```python
from build123d import *

# Parameters (mm, degrees)
SKETCH_1_W          = 7
SKETCH_1_H          = 7
EXTRUDE_1_DEPTH     = 51
SKETCH_2_W          = 3.5
SKETCH_2_H          = 7
EXTRUDE_2_DEPTH     = 7
SKETCH_3_W          = 3.5
SKETCH_3_H          = 7
EXTRUDE_3_DEPTH     = 7
FILLET_1_R          = 3.5
SKETCH_4_R          = 1.55
CUT_EXTRUDE_1_DEPTH = 3.5
CUT_EXTRUDE_2_DEPTH = 3.5
FILLET_2_R          = 2


with BuildPart() as part:
    # 草图1 → 凸台-拉伸1 (new body)
    with BuildSketch(Plane.XY):
        Rectangle(SKETCH_1_W, SKETCH_1_H)
    extrude(amount=EXTRUDE_1_DEPTH)

    # 草图2 → 凸台-拉伸2 (add)
    with BuildSketch(Plane.XY.offset(51)):
        with Locations((1.75, 0)):
            Rectangle(SKETCH_2_W, SKETCH_2_H)
    extrude(amount=EXTRUDE_2_DEPTH)

    # 草图3 → 凸台-拉伸3 (add)
    with BuildSketch(Plane(origin=(0, 0, 0), x_dir=(-1, 0, 0), z_dir=(0, 0, -1))):
        with Locations((-1.75, 0)):
            Rectangle(SKETCH_3_W, SKETCH_3_H)
    extrude(amount=EXTRUDE_3_DEPTH)

    # 圆角1
    fillet_1_edges = [part.edges().sort_by_distance(p)[0] for p in [
        (1.75, -3.5, 58),
        (1.75, 3.5, 58),
        (1.75, 3.5, -7),
        (1.75, -3.5, -7),
    ]]
    fillet(fillet_1_edges, radius=FILLET_1_R - 0.0001)  # a hair under: the kernel refuses the full size

    # 草图4 → 切除-拉伸1 (cut)
    with BuildSketch(Plane.ZY):
        with Locations((54.5, 0)):
            Circle(SKETCH_4_R)
        with Locations((-3.5, 0)):
            Circle(SKETCH_4_R)
    extrude(amount=-CUT_EXTRUDE_1_DEPTH, mode=Mode.SUBTRACT)

    # 草图5 → 切除-拉伸2 (cut)
    with BuildSketch(Plane.ZY.offset(3.5)):
        Polygon((0, 3.5), (7, -3.5), (0, -3.5), align=None)
    extrude(amount=-CUT_EXTRUDE_2_DEPTH, mode=Mode.SUBTRACT)

    # 圆角2
    fillet_2_edges = [part.edges().sort_by_distance(p)[0] for p in [
        (3.5, -3.5, 25.5),
        (-3.5, -3.5, 29),
        (3.5, 3.5, 25.5),
        (-3.5, 3.5, 25.5),
    ]]
    fillet(fillet_2_edges, radius=FILLET_2_R)


solid = part.part
```
Model file for the job. Use its own axes, mm. A direction names the side the tool comes from. Give positions to 0.01 mm unless a question says otherwise; leave off trailing zeros. Loops run counter-clockwise (first coordinate to the right, second up) from the corner with the lowest first, then second, coordinate; pieces in that order, holes last. Notation, with made-up numbers: M 18,76 L 74,76 A23 cw 74,91 Z; hole C 33,-14 d11. An arc over 180 degrees is marked long. Use one line per item in the form item = value.
Item 1: Which spindle directions (+Z, -Z, +X, -X, +Y, -Y) get a long thin tool onto all of the face, cutting with end or side? Do faces 1 (the flat face through (-2, 0, 51)), 2 (the cylindrical face through (0.74, -2.5, -5.95)), 3 (the flat face through (-1.8, 0, 3.5)). Say none if no direction does.
Filled in:
face_1 = +Z, -X, +Y, -Y
face_2 = -Z, +X, -X, -Y
face_3 = -Z, -X, -Y
Item 2: Slice it at B-B on y = -0.75. Give the number of separate pieces and of enclosed holes in the cut face, and give its area (3 significant figures).
Filled in:
separate_pieces = 3
enclosed_holes = 0
area = 370 mm^2
Item 3: Drill centre lines: L1, parallel to Y at x = 1.4, z = 54.5; L2, parallel to Z at x = 0.75, y = 0.5; L3, parallel to Z at x = 1, y = -0.75. Where is each one in solid material? Low to high.
Filled in:
L1 = -3.5 to -1.55, 1.55 to 3.5
L2 = -6.96 to -4.97, -2.03 to 53.03, 55.97 to 57.96
L3 = -6.92 to -4.86, -2.14 to 53.14, 55.86 to 57.92
Item 4: Flat gauge pins, fed straight in: pin 1 Ø1.8 at (x, y) = (-2, 1.5) entering from +Z; pin 2 Ø1 at (y, z) = (3, 13.5) entering from -X. Where does each tip first touch, or does it go through?
Filled in:
pin_1 = 51
pin_2 = -3.23
Item 5: Two-plate mould, pull along Z, no slides. Class faces 4 (the cylindrical face through (1.726, -0.594, 55.932)), 5 (the cylindrical face through (1.73, 0.07, -5.05)), 6 (the flat face through (0, -1, -1)), 7 (the cylindrical face through (0.76, 2.45, 57)): released by +Z, released by -Z, zero draft, split by the parting line, or undercut.
Filled in:
face_4 = undercut
face_5 = undercut
face_6 = zero draft
face_7 = released by +Z
Item 6: Slice it at A-A on z = 47. List the corners of the cut face in (x, y), and give its area (3 significant figures).
Filled in:
outline = M -3.5,-1.5 A2 ccw -1.5,-3.5 L 1.5,-3.5 A2 ccw 3.5,-1.5 L 3.5,1.5 A2 ccw 1.5,3.5 L -1.5,3.5 A2 ccw -3.5,1.5 Z
area = 45.6 mm^2
